For this review, take the finished solid that the model builds, in its own axes (mm). A direction names the side the tool comes from. Coordinates: 2 decimals unless noted, no trailing zeros. Write each loop counter-clockwise with the first axis right and the second up, starting at its lowest first coordinate (ties: lowest second). Pieces come first, ordered by that corner, then holes.
Autodesk Inventor part; units mm, degrees
ref_plane "YZ Plane" through (0, 0, 0) normal (1, 0, 0) x (0, 1, 0)
ref_plane "XZ Plane" through (0, 0, 0) normal (0, 1, 0) x (-1, 0, 0)
ref_plane "XY Plane" through (0, 0, 0) normal (0, 0, 1) x (1, 0, 0)
sketch "Sketch1" plane through (0, 0, 0) normal (0, 0, 1) x (1, 0, 0)
  circle A0 centre (0, 0) radius 3.2
  line L0 (-3.1984, 0.1) -> (-10.25, 0.1)
  line L1 (-10.25, 0.1) -> (-10.25, 3.6)
  line L2 (-10.25, 3.6) -> (-5.6507, 3.6)
  arc A1 (5.6507, 3.6) -> (-5.6507, 3.6) centre (0, 0) ccw
  line L3 (5.6507, 3.6) -> (10.25, 3.6)
  line L4 (10.25, 3.6) -> (10.25, 2.7012)
  line L5 (10.25, 2.7012) -> (10.25, 0.1)
  line L6 (10.25, 0.1) -> (6.1992, 0.1)
  line L7 (6.1992, 0.1) -> (3.1984, 0.1)
  dimension "d0" = 6.4
  dimension "d1" = 0.1
  dimension "d2" = 3.5
  dimension "d3" = 3.5
  dimension "d4" = 10.25
  dimension "d5" = 10.25
extrude "Extrusion1" add sketch "Sketch1" along normal blind 5.5 contours A0 L0 L1 L2 A1 L3 L4 L5 L6 L7
sketch "Sketch2" plane through (-10.25, 3.6, 0) normal (0, 1, 0) x (1, 0, 0)
  circle A0 centre (2.75, -2.75) radius 3.5
  circle A1 centre (17.75, -2.75) radius 3.5
  line L0 (0, 0) -> (0, -5.5)
  line L1 (20.5, 0) -> (20.5, -5.5)
  point P0 (10.25, 0)
  point P1 (0, -2.75)
  dimension "d8" = 15
  dimension "d9" = 2.75
  dimension "d10" = 2.75
  dimension "d11" = 7
extrude "Extrusion2" cut sketch "Sketch2" along normal through all
sketch "Sketch3" plane through (-10.25, 3.6, 5.5) normal (0, 1, 0) x (1, 0, 0)
  arc A0 (4.9151, 0) -> (4.9151, 5.5) centre (2.75, 2.75) ccw
  circle A1 centre (2.75, 2.75) radius 1.55
  arc A2 (15.5849, 5.5) -> (15.5849, 0) centre (17.75, 2.75) ccw
  circle A3 centre (17.75, 2.75) radius 1.55
  line L0 (4.9151, 5.5) -> (15.5849, 5.5)
  line L1 (0, 5.5) -> (0, 0)
  line L2 (4.9151, 0) -> (0, 0)
  arc A4 (4.9151, 0) -> (4.9151, 5.5) centre (2.75, 2.75) ccw
  line L3 (4.9151, 5.5) -> (0, 5.5)
  line L4 (20.5, 5.5) -> (20.5, 0)
  line L5 (20.5, 5.5) -> (15.5849, 5.5)
  arc A5 (15.5849, 5.5) -> (15.5849, 0) centre (17.75, 2.75) ccw
  line L6 (20.5, 0) -> (15.5849, 0)
  circle A6 centre (17.75, 2.75) radius 2.75
  line L7 (20.5, 5.5) -> (15.5849, 5.5)
  circle A7 centre (2.75, 2.75) radius 2.75
  point P0 (10.25, 5.5)
  point P1 (15.5849, 0)
  point P2 (2.75, 0)
  point P3 (0, 2.75)
  point P4 (2.75, 5.5)
  point P5 (20.5, 2.75)
  point P6 (17.75, 0)
  point P7 (17.75, 5.5)
  dimension "d14" = 3.1
extrude "Extrusion3" cut sketch "Sketch3" against normal through all contours L2 L1 A7 | A7 L1 L3 | L5 L4 A6 | A6 L4 L6 | A1 | A3
equation "\"d3\" = d2"
equation "\"d9\" = d10"
properties part number "suction_clip_2_top"
Q1. Tool access review of faces 1 (the flat face through (5.7, 3.6, 2.7)), 2 (the cylindrical face through (-4, 4.3, 2.7)), 3 (the cylindrical face through (10.25, 1.87, 2.81)): name each direction out of +Z, -Z, +X, -X, +Y, -Y from which nothing blocks a thin tool from reaching the whole face with its end or side.
Ans:
face 1: +X, +Y
face 2: -X, +Y
face 3: +X, +Y, -Y
Q2. For probe 1 along X at (y, z) = (1, 2.9); probe 2 along X at (y, z) = (2, 2.7); probe 3 along Z at (x, y) = (-7.5, 2.2), list the stretches that pass through material, from the lowest coordinate up.
Ans:
probe 1: x = -10.25 to -9.04, -5.96 to -3.04, 3.04 to 5.96, 9.04 to 10.25
probe 2: x = -10.25 to -9.05, -5.95 to -2.5, 2.5 to 5.95, 9.05 to 10.25
probe 3: z = 0 to 1.2, 4.3 to 5.5
Q3. Add section D-D (z = 4). State the section outline as (x, y) points.
Ans:
outline: (-9.95, 0.1) - (-8.42, 0.1) - (-8.42, 3.6) - (-9.95, 3.6) - close; (-6.58, 0.1) - (-3.2, 0.1) arc R3.2 cw to (3.2, 0.1) - (6.58, 0.1) - (6.58, 3.6) - (4.23, 3.6) - (4.23, 5.2) arc R6.7 ccw to (-4.23, 5.2) - (-4.23, 3.6) - (-6.58, 3.6) - close; (8.42, 0.1) - (9.95, 0.1) - (9.95, 3.6) - (8.42, 3.6) - close
Q4. Add section C-C (x = -7). State the section outline as (y, z) points.
Ans:
outline: (0.1, 0) - (3.6, 0) - (3.6, 1.28) - (0.1, 1.28) - close; (0.1, 4.22) - (3.6, 4.22) - (3.6, 5.5) - (0.1, 5.5) - close
Q5. Draft analysis for pull direction X (two halves, no side actions). For faces 4 (the cylindrical face through (-0.1, 3.2, 2.7)), 5 (the cylindrical face through (8.215, 1.874, 4.125)), 6 (the cylindrical face through (-0.1, 6.7, 2.7)), 7 (the flat face through (-0.1, 3.4, 5.5)), state which applies: +X half, -X half, draft (parallel to the pull), parting line (faces both ways), or undercut.
Ans:
face 4: undercut
face 5: undercut
face 6: parting line
face 7: draft
Q6. Add section A-A (y = 1.5). State the section outline as (x, z) points.
Ans:
outline: (-7.5, 0) - (-2.83, 0) - (-2.83, 5.5) - (-7.5, 5.5) arc R2.75 ccw to start; (2.83, 0) - (7.5, 0) arc R2.75 ccw to (7.5, 5.5) - (2.83, 5.5) - close; hole circle Ø3.1 at (-7.5, 2.75); hole circle Ø3.1 at (7.5, 2.75)
Q7. Add section B-B (z = 2.55). State the section outline as (x, y) points, then the cut area to 3 significant figures.
Ans:
outline: (-10.24, 0.1) - (-9.04, 0.1) - (-9.04, 3.6) - (-10.24, 3.6) - close; (-5.96, 0.1) - (-3.2, 0.1) arc R3.2 cw to (3.2, 0.1) - (5.96, 0.1) - (5.96, 3.6) - (4.01, 3.6) - (4.01, 5.37) arc R6.7 ccw to (-4.01, 5.37) - (-4.01, 3.6) - (-5.96, 3.6) - close; (9.04, 0.1) - (10.24, 0.1) - (10.24, 3.6) - (9.04, 3.6) - close
area: 56.2 mm2
Q8. Clearance check with flat-ended pins moving along their axes: pin 1 Ø1 at (y, z) = (5, 2.5) entering from +X; pin 2 Ø1 at (x, z) = (0.5, 3) entering from -Y; pin 3 Ø1 at (y, z) = (1, 4) entering from +X; pin 4 Ø2.5 at (x, z) = (7.5, 2.75) entering from -Y. State where each tip first meets the part, or that it passes through.
Ans:
pin 1: stops at x = 4.08
pin 2: stops at y = 3.04
pin 3: stops at x = 10.15
pin 4: passes through
